Can you work these out from the model? Positions are in its coordinate system, mm. A direction names the side the tool comes from. Give positions to 0.01 mm unless a question says otherwise; leave off trailing zeros. Loops run counter-clockwise (first coordinate to the right, second up) from the corner with the lowest first, then second, coordinate; pieces in that order, holes last. Notation, with made-up numbers: (-19.5, -6.5) -> (32.5, -6.5) arc R20 cw to (32.5, 26.5) -> close; hole circle Ø5 at (89.25, 65). An arc over 180 degrees is marked (long way). Use CSV: the item, a comma, the result in double quotes.
from build123d import *

# Parameters (mm, degrees)
F0_R     = 50.8
F1_DEPTH = 19.05
F2_R     = 25.4
F3_DEPTH = 57.15
F3_TAPER = 5
F4_R     = 12.7
F5_DEPTH = 254
F6_R     = 12.7


# Not quite as in the source:
# - the program builds the solid bodies; features that only make, move or delete a surface that nothing else refers to are left out


with BuildPart() as f1:
    # F0 (on Front) → F1 (new body)
    with BuildSketch(Plane.XZ):
        Circle(F0_R)
    extrude(amount=F1_DEPTH)

    # F2 (on face) → F3 (join)
    with BuildSketch(Plane.XZ.offset(19.05)):
        with Locations((0, -12.7)):
            Circle(F2_R)
    extrude(amount=F3_DEPTH, taper=F3_TAPER)

    # F4 (on face) → F5 (join)
    with BuildSketch(Plane.XZ.offset(76.2)):
        with Locations((0, -12.7)):
            Circle(F4_R)
    extrude(amount=F5_DEPTH)

    # F8: sweep along a path in F7
    with BuildLine(Plane.YZ) as f8_path:
        ThreePointArc((-330.2, -12.7), (-366.1210244843, -27.5789755157), (-381, -63.5))
    # F6 (on face) → F8 (sweep)
    with BuildSketch(Plane.XZ.offset(330.2)):
        with Locations((0, -12.7)):
            Circle(F6_R)
    sweep(path=f8_path.line)


solid = f1.part
(1) If we section it at B-B, the plane y = -170: Write out the boundary of the cut face in (x, z).
Answer sheet:
outline,"circle Ø25.4 at (0, -12.7)"
(2) Will this pin go through, and if not, where does the flat tip stop? pin 1 Ø10 at (y, z) = (-331.5, -25) entering from +X.
Answer sheet:
pin 1,"stops at x = 10.41"
(3) If I drill on L1, parallel to Y at x = -26.5, z = -2; L2, parallel to Y at x = 15.5, z = -19; L3, parallel to Y at x = -4, z = -38.5, over which ranges is the centre line in solid material (lowest first)? Write a range as from..to.
Answer sheet:
L1,"y = -19.05..0"
L2,"y = -76.2..0"
L3,"y = -387.87..-359.8, -19.05..0"
(4) If we section it at C-C, the plane y = -26: Write out the boundary of the cut face in (x, z).
Answer sheet:
outline,"circle Ø49.58 at (0, -12.7)"
(5) If we section it at A-A, the plane x = 0: Write out the boundary of the cut face in (y, z), then the cut area to 3 significant figures.
Answer sheet:
outline,"(-393.7, -63.5) -> (-368.3, -63.5) arc R38.1 cw to (-330.2, -25.4) -> (-76.2, -25.4) -> (-76.2, -33.1) -> (-19.05, -38.1) -> (-19.05, -50.8) -> (0, -50.8) -> (0, 50.8) -> (-19.05, 50.8) -> (-19.05, 12.7) -> (-76.2, 7.7) -> (-76.2, 0) -> (-330.2, 0) arc R63.5 ccw to start"
area,"13,000 mm2"
(6) If we section it at D-D, the plane x = -36: Write out the boundary of the cut face in (y, z).
Answer sheet:
outline,"(-19.05, -35.84) -> (0, -35.84) -> (0, 35.84) -> (-19.05, 35.84) -> close"
(7) Which directions (+Z, -Z, +X, -X, +Y, -Y) give clear straight access to the entire face, cutting with the end or side of a thin tool? Please do faces 1 (the face through (9, -76.2, -3)), 2 (the face through (0, -381, -63.5)).
Answer sheet:
face 1,"none"
face 2,"-Z, +X, -X, +Y, -Y"
